Here's how the part is built. I have some questions about the finished solid (model axes, mm). Face numbers are marked on the shaded views. A direction names the side the tool comes from. Give positions to 0.01 mm unless a question says otherwise; leave off trailing zeros. Write each loop counter-clockwise with the first axis right and the second up, starting at its lowest first coordinate (ties: lowest second). Pieces come first, ordered by that corner, then holes. Notation, with made-up numbers: (58, 74.5) - (77, 74.5) arc R29 cw to (77, 96.5) - close; hole circle Ø9 at (87.25, -9). An arc over 180 degrees is marked (long way). Use a Markdown table: item, result.
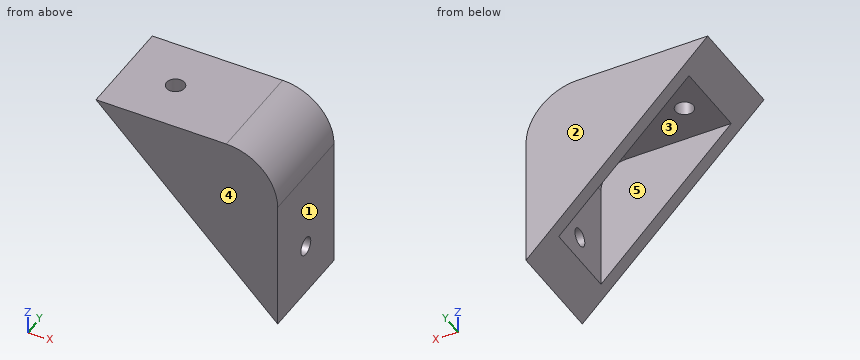
```python
from build123d import *

# Parameters (mm, degrees)
BOSS_EXTRUDE1_DEPTH = 10
FILLET1_R           = 10
CUT_EXTRUDE1_START  = -5
SKETCH5_W           = 25.355339059
SKETCH5_H           = 15
CUT_EXTRUDE1_DEPTH  = 31.355339059
CUT_EXTRUDE3_START  = -5
SKETCH6_W           = 25.355339059
SKETCH6_H           = 15
CUT_EXTRUDE3_DEPTH  = 31.355339059
SKETCH8_W           = 5
SKETCH8_H           = 15
SKETCH9_R           = 1.75
CUT_EXTRUDE4_DEPTH  = 6
SKETCH10_R          = 1.75
CUT_EXTRUDE5_DEPTH  = 6


with BuildPart() as part:
    # Sketch1 → Boss-Extrude1 (new body, symmetric)
    with BuildSketch(Plane(origin=(0, 0, 0), x_dir=(1, 0, 0), z_dir=(0, 1, 0))):
        Polygon((0, 0), (0, 35.355339059), (-35.355339059, 0), align=None)
    extrude(amount=BOSS_EXTRUDE1_DEPTH, both=True)

    # Fillet1
    fillet1_edges = [part.edges().sort_by_distance(p)[0] for p in [
        (0, 0, 0),
    ]]
    fillet(fillet1_edges, radius=FILLET1_R)

    # Sketch5 → Cut-Extrude1 (cut, through all)
    with BuildSketch(Plane.XY.offset(CUT_EXTRUDE1_START)):
        with Locations((-22.67766953, 0)):
            Rectangle(SKETCH5_W, SKETCH5_H)
    extrude(amount=-CUT_EXTRUDE1_DEPTH, mode=Mode.SUBTRACT)

    # Sketch6 → Cut-Extrude3 (cut, through all)
    with BuildSketch(Plane(origin=(0, 0, 0), x_dir=(0, 0, -1), z_dir=(1, 0, 0)).offset(CUT_EXTRUDE3_START)):
        with Locations((22.67766953, 0)):
            Rectangle(SKETCH6_W, SKETCH6_H)
    extrude(amount=-CUT_EXTRUDE3_DEPTH, mode=Mode.SUBTRACT)

    # Sketch8 → Cut-Revolve2 (revolve, cut)
    with BuildSketch(Plane(origin=(0, 0, -10), x_dir=(-1, 0, 0), z_dir=(0, 0, -1))):
        with Locations((7.5, 0)):
            Rectangle(SKETCH8_W, SKETCH8_H)
    revolve(axis=Axis((-10, -7.5, -10), (0, 1, 0)), mode=Mode.SUBTRACT)

    # Sketch9 → Cut-Extrude4 (cut, through all)
    with BuildSketch(Plane.ZY.offset(5)):
        with Locations((-25.355339059, 0)):
            Circle(SKETCH9_R)
    extrude(amount=-CUT_EXTRUDE4_DEPTH, mode=Mode.SUBTRACT)

    # Sketch10 → Cut-Extrude5 (cut, through all)
    with BuildSketch(Plane(origin=(0, 0, -5), x_dir=(-1, 0, 0), z_dir=(0, 0, -1))):
        with Locations((25.355339059, 0)):
            Circle(SKETCH10_R)
    extrude(amount=-CUT_EXTRUDE5_DEPTH, mode=Mode.SUBTRACT)


solid = part.part
```
Item 1: For the marked faces 4 and 5, which set-ups out of +Z, -Z, +X, -X, +Y, -Y let a thin tool reach every point of the face, with its end or its side?
Values:
| item | result |
|---|---|
| face 4 | +Z, -Z, +X, -X, -Y |
| face 5 | -Z, -X |
Item 2: Will these pins go through, and if not, where does the flat tip stop? pin 1 Ø2 at (x, y) = (-24.5, 4.5) entering from -Z; pin 2 Ø6 at (x, y) = (-5.5, 0.5) entering from +Z; pin 3 Ø2 at (x, y) = (-25.36, 0) entering from +Z; pin 4 Ø4 at (x, y) = (-8, -3.5) entering from -Z.
Values:
| item | result |
|---|---|
| pin 1 | stops at z = -5 |
| pin 2 | stops at z = -0.11 |
| pin 3 | passes through |
| pin 4 | stops at z = -7 |
Item 3: If we section it at B-B, the plane y = -6.5: Write out the boundary of the cut face in (x, z).
Values:
| item | result |
|---|---|
| outline | (-35.36, 0) - (-30.36, -5) - (-10, -5) arc R5 cw to (-5, -10) - (-5, -30.36) - (0, -35.36) - (0, -10) arc R10 ccw to (-10, 0) - close |
Item 4: I need wall thicknesses on line 1 along Y through (x, z) = (-12, -5.5); line 2 along X through (y, z) = (0.5, -18.5). Which ranges of each line are inside material? Lowest first, please. Write a range as [from, to].
Values:
| item | result |
|---|---|
| line 1 | y = [-10, -7.5], [7.5, 10] |
| line 2 | x = [-5, 0] |
Item 5: If we section it at A-A, the plane y = 0: Write out the boundary of the cut face in (x, z), plus the area to 3 significant figures.
Values:
| item | result |
|---|---|
| outline | (-35.36, 0) - (-30.36, -5) - (-27.11, -5) - (-27.11, 0) - close; (-23.61, -5) - (-10, -5) arc R5 cw to (-5, -10) - (-5, -23.61) - (0, -23.61) - (0, -10) arc R10 ccw to (-10, 0) - (-23.61, 0) - close; (-5, -30.36) - (0, -35.36) - (0, -27.11) - (-5, -27.11) - close |
| area | 252 mm2 |
Item 6: If we section it at D-D, the plane z = -22: Write out the boundary of the cut face in (x, y), plus the area to 3 significant figures.
Values:
| item | result |
|---|---|
| outline | (-13.36, -10) - (0, -10) - (0, 10) - (-13.36, 10) - (-13.36, 7.5) - (-5, 7.5) - (-5, -7.5) - (-13.36, -7.5) - close |
| area | 142 mm2 |
Item 7: If we section it at C-C, the plane x = -2: Write out the boundary of the cut face in (y, z), plus the area to 3 significant figures.
Values:
| item | result |
|---|---|
| outline | (-10, -33.36) - (10, -33.36) - (10, -4) - (-10, -4) - close; hole circle Ø3.5 at (0, -25.36) |
| area | 577 mm2 |
Item 8: Thinking about a two-plate mould opening in Y: for the marked faces 1, 2 and 3, which applies, +Y half, -Y half, draft (parallel to the pull), parting line (faces both ways), or undercut?
Values:
| item | result |
|---|---|
| face 1 | draft |
| face 2 | +Y half |
| face 3 | undercut |
